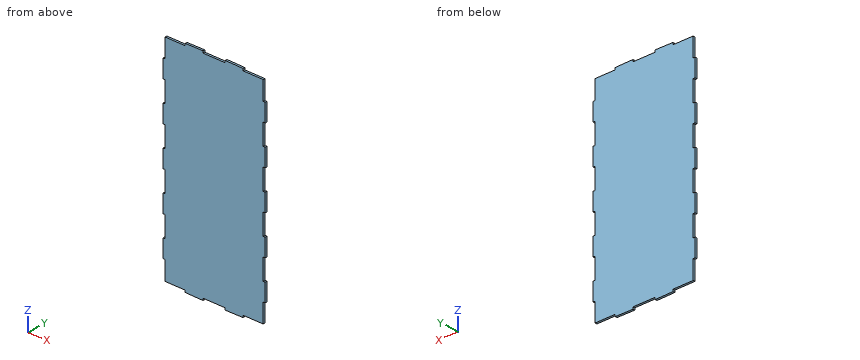
```python
from build123d import *

# Parameters (mm, degrees)
BOSS_EXTRUDE1_DEPTH = 5.7


with BuildPart() as part:
    # Sketch1 → Boss-Extrude1 (new body)
    with BuildSketch(Plane(origin=(0, 0, 0), x_dir=(1, 0, 0), z_dir=(0, 1, 0))):
        Polygon((31.75, 299.891703858), (-31.75, 299.891703858), (-31.75, 305.591703858), (-82.54382924, 304.79992666), (-82.55, 299.09993), (-140.35, 299.09993), (-140.35, 245.5366), (-146.05, 245.5366), (-146.05, 194.7366), (-140.35, 194.7366), (-140.35, 135.47), (-146.05, 135.47), (-146.05, 84.67), (-140.35, 84.67), (-140.35, 25.4), (-146.05, 25.4), (-146.05, -25.4), (-140.35, -25.4), (-140.35, -84.67), (-146.05, -84.67), (-146.05, -135.47), (-140.35, -135.47), (-140.35, -194.7366), (-146.05, -194.7366), (-146.05, -245.5366), (-140.35, -245.5366), (-140.35, -299.09993), (-82.55, -299.09993), (-82.54382924, -304.79992666), (-31.75, -305.591703858), (-31.75, -299.891703858), (31.75, -299.891703858), (31.75, -305.591703858), (82.54382924, -304.79992666), (82.55, -299.09993), (140.35, -299.09993), (140.35, -245.5366), (146.05, -245.5366), (146.05, -194.7366), (140.35, -194.7366), (140.35, -135.47), (146.05, -135.47), (146.05, -84.67), (140.35, -84.67), (140.35, -25.4), (146.05, -25.4), (146.05, 25.4), (140.35, 25.4), (140.35, 84.67), (146.05, 84.67), (146.05, 135.47), (140.35, 135.47), (140.35, 194.7366), (146.05, 194.7366), (146.05, 245.5366), (140.35, 245.5366), (140.35, 299.09993), (82.55, 299.09993), (82.54382924, 304.79992666), (31.75, 305.591703858), align=None)
    extrude(amount=BOSS_EXTRUDE1_DEPTH)


solid = part.part
```
Check sheet for the modelled part. Datum: model origin and axes. Units: mm. Coordinates: 2 decimals unless noted, no trailing zeros. Order: outer loops, then holes, each group sorted by start corner. A loop starts at its lowest first (then second) coordinate and runs counter-clockwise, first axis right, second up. Notation, with made-up numbers: (44.25, 68) -> (83.25, 68) arc R17 ccw to (83.25, 84) -> close; hole circle Ø11 at (0, 13). An arc over 180 degrees is marked (long way). Write item = value, one per line. Start each with the question number.
1) Material ranges on L1, parallel to Z at x = 5.5, y = 5.25; L2, parallel to Z at x = -91.5, y = 2; L3, parallel to X at y = 1.25, z = 64.5, recorded low to high.
2) Cross-section at A-A (x = -7). Enter the section's corners in (y, z), then the cut area to 3 significant figures.
3) Cross-section at B-B (z = -69). Enter the section's corners in (x, y).
4) Go/stop test with flat-tipped pins: P1, Ø3, axis at x = 144.5, y = 3, coming from the +Z side; P2, Ø1.7, axis at x = 11.5, y = 3.5, coming from the -Z side; P3, Ø3, axis at y = 3.5, z = 161, coming from the +X side. Record where each tip stops, or that it passes through.
Ans:
q1.L1 = -299.89 to 299.89
q1.L2 = -299.1 to 299.1
q1.L3 = -140.35 to 140.35
q2.outline = (0, -299.89) -> (5.7, -299.89) -> (5.7, 299.89) -> (0, 299.89) -> close
q2.area = 3,420 mm²
q3.outline = (-140.35, 0) -> (140.35, 0) -> (140.35, 5.7) -> (-140.35, 5.7) -> close
q4.P1 = 245.54
q4.P2 = -299.89
q4.P3 = 140.35
